Geometry: final body of the model. Coordinates: model frame, mm. Give positions to 0.01 mm unless a question says otherwise; leave off trailing zeros. Write each loop counter-clockwise with the first axis right and the second up, starting at its lowest first coordinate (ties: lowest second). Pieces come first, ordered by that corner, then holes.
Autodesk Inventor part; units mm, degrees
ref_plane "YZ Plane" through (0, 0, 0) normal (1, 0, 0) x (0, 1, 0)
ref_plane "XZ Plane" through (0, 0, 0) normal (0, 1, 0) x (-1, 0, 0)
ref_plane "XY Plane" through (0, 0, 0) normal (0, 0, 1) x (1, 0, 0)
sketch "스케치2" plane through (0, 0, 0) normal (0, 1, 0) x (-1, 0, 0)
  line L0 (0, 45) -> (38.9711, 22.5)
  line L1 (38.9711, 22.5) -> (38.9711, -22.5)
  line L2 (38.9711, -22.5) -> (0, -45)
  line L3 (0, -45) -> (-38.9711, -22.5)
  line L4 (-38.9711, -22.5) -> (-38.9711, 22.5)
  line L5 (-38.9711, 22.5) -> (0, 45)
  line L6 (0, 50.7735) -> (43.9711, 25.3868)
  line L7 (43.9711, 25.3868) -> (43.9711, -25.3868)
  line L8 (43.9711, -25.3868) -> (0, -50.7735)
  line L9 (0, -50.7735) -> (-43.9711, -25.3868)
  line L10 (-43.9711, -25.3868) -> (-43.9711, 25.3868)
  line L11 (-43.9711, 25.3868) -> (0, 50.7735)
  line L12 (-43.9711, 25.3868) -> (-38.9711, 22.5)
  line L13 (-38.9711, -22.5) -> (-43.9711, -25.3868)
  point P0 (0, 0)
  point P1 (0, 0)
  dimension "d0" = 45
  dimension "d1" = 5
extrude "돌출1" add sketch "스케치2" along normal blind 80 contours L4 L13 L10 L12
sketch "스케치3" plane through (38.9711, 0, -22.5) normal (-1, 0, 0) x (0, 0, 1)
  line L0 (0, 0) -> (45, 0) construction
  circle A0 centre (22.5, 24.4) radius 2.6
  point P0 (22.5, 0)
  point P1 (22.5, 0)
  dimension "d4" = 5.2
  dimension "d5" = 24.4
extrude "돌출2" cut sketch "스케치3" against normal through all
sketch "스케치4" plane through (0, 80, 0) normal (0, 1, 0) x (1, 0, 0)
  line L0 (38.9711, 22.5) -> (38.9711, -22.5) construction
  circle A0 centre (41.4711, 0) radius 2.5
  point P0 (0, 0)
  dimension "d8" = 5
extrude "돌출3" add sketch "스케치4" along normal blind 5
sketch "스케치5" plane through (43.9711, 0, 25.3868) normal (1, 0, 0) x (0, 0, -1)
  line L0 (50.7735, 0) -> (50.7735, 80) construction
  line L1 (25.3868, 80) -> (50.7735, 80) construction
  line L2 (0, 0) -> (0, 80) construction
  circle A0 centre (25.3868, 60) radius 2.6
  circle A1 centre (13.3868, 60) radius 2.6
  circle A2 centre (37.3868, 60) radius 2.6
  line L3 (0, 60) -> (50.7735, 60)
  point P0 (25.3868, 0)
  dimension "d11" = 20
  dimension "d12" = 0
  dimension "d13" = 0
  dimension "d14" = 0
  dimension "d15" = 12
  dimension "d16" = 12
  dimension "d17" = 5.2
  dimension "d18" = 5.2
  dimension "d19" = 5.2
extrude "돌출4" cut sketch "스케치5" against normal through all
chamfer "모따기1" distance 1 angle 45 5 edges at (38.9711, 85, 0) (38.9711, 60, -9.4) (38.9711, 60, 2.6) (38.9711, 60, 14.6) (38.9711, 24.4, -2.6)
properties part number "col_face"
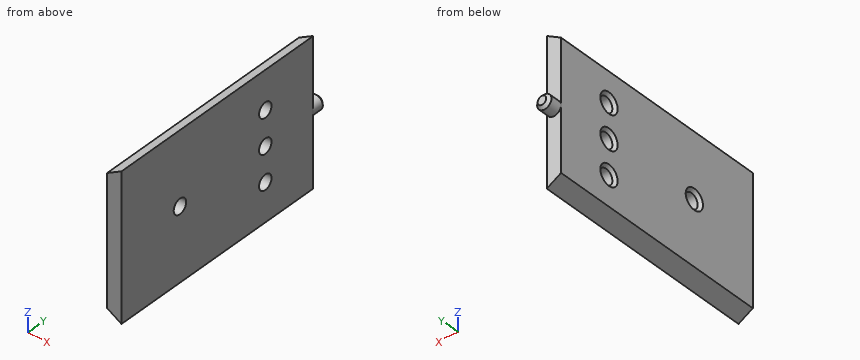
Q1. Section C-C on y = 60. Output: boundary loops of the cut face in (x, z).
Filled sheet:
outline: (38.97, -22.5) - (43.97, -25.39) - (43.97, -14.6) - (39.97, -14.6) - (38.97, -15.6) - close; (38.97, -8.4) - (39.97, -9.4) - (43.97, -9.4) - (43.97, -2.6) - (39.97, -2.6) - (38.97, -3.6) - close; (38.97, 3.6) - (39.97, 2.6) - (43.97, 2.6) - (43.97, 9.4) - (39.97, 9.4) - (38.97, 8.4) - close; (38.97, 15.6) - (39.97, 14.6) - (43.97, 14.6) - (43.97, 25.39) - (38.97, 22.5) - close
Q2. Section A-A on y = 24.4. Output: boundary loops of the cut face in (x, z), plus the area to 3 significant figures.
Filled sheet:
outline: (38.97, -22.5) - (43.97, -25.39) - (43.97, -2.6) - (39.97, -2.6) - (38.97, -3.6) - close; (38.97, 3.6) - (39.97, 2.6) - (43.97, 2.6) - (43.97, 25.39) - (38.97, 22.5) - close
area: 212 mm2
Q3. Section D-D on z = 5.5. Output: boundary loops of the cut face in (x, y), plus the area to 3 significant figures.
Filled sheet:
outline: (38.97, 0) - (43.97, 0) - (43.97, 80) - (38.97, 80) - close
area: 400 mm2
Q4. Pin query (flat end, axial travel): P1, Ø1.5, axis at x = 40, z = 12, coming from the -Y side. Return the tip coordinate at first contact, or that it passes through.
Filled sheet:
P1: stops at y = 0
Q5. Section B-B on z = 12. Output: boundary loops of the cut face in (x, y), plus the area to 3 significant figures.
Filled sheet:
outline: (38.97, 0) - (43.97, 0) - (43.97, 57.4) - (39.97, 57.4) - (38.97, 56.4) - close; (38.97, 63.6) - (39.97, 62.6) - (43.97, 62.6) - (43.97, 80) - (38.97, 80) - close
area: 373 mm2
Q6. Ray query, line 1 along Y through (x, z) = (41.1, 0); line 2 along Z through (x, y) = (41.35, 60); line 3 along Y through (x, z) = (41.45, -12). Return the intervals inside material, ascending.
Filled sheet:
line 1: y = 0 to 21.8, 27 to 57.4, 62.6 to 85
line 2: z = -23.87 to -14.6, -9.4 to -2.6, 2.6 to 9.4, 14.6 to 23.87
line 3: y = 0 to 57.4, 62.6 to 80
